Autodesk Fusion 360 part; units mm, degrees
sketch "Sketch1" plane through (0, 0, 0) normal (0, 1, 0) x (1, 0, 0)
  line L0 (0, 80) -> (-33.9737, 46.7608)
  line L1 (0, 80) -> (33.9737, 46.7608)
  line L2 (-76.0845, 24.7214) -> (-33.9737, 46.7608)
  line L3 (-76.0845, 24.7214) -> (-54.9706, -17.861)
  line L4 (-47.0228, -64.7214) -> (-54.9706, -17.861)
  line L5 (-47.0228, -64.7214) -> (0, -57.7996)
  line L6 (47.0228, -64.7214) -> (0, -57.7996)
  line L7 (47.0228, -64.7214) -> (54.9706, -17.861)
  line L8 (76.0845, 24.7214) -> (54.9706, -17.861)
  line L9 (76.0845, 24.7214) -> (33.9737, 46.7608)
  circle A0 centre (0, 0) radius 25
  dimension "d35" = 50
extrude "Extrude1" add sketch "Sketch1" along normal blind 25 contours L0 L1 L2 L3 L4 L5 L6 L7 L8 L9 | A0 makes body 1
shell "Shell1" thickness 5 outward yes removed faces 1 at (11.3246, 25, -3.6796) on bodies 1
extrude "Extrude2" add 1 faces at (-65.2553, 25, -34.1513) along direction (0, 1, 0) blind 5 separate body on bodies 1 makes body 2
extrude "Extrude3" add sketch "Sketch1" along normal blind 30 separate body contours L0 L1 L2 L3 L4 L5 L6 L7 L8 L9 | A0 makes body 3
extrude "Extrude4" cut 1 faces at (11.3246, 0, -3.6796) along direction (0, 1, 0) blind 25 on bodies 3 bodies 3
sketch "Sketch2" plane through (0, 30, 0) normal (0, 1, 0) x (-1, 0, 0)
  line L0 (-47.0228, 64.7214) -> (-54.9706, 17.861)
  line L1 (-54.9706, 17.861) -> (-76.0845, -24.7214)
  line L2 (-76.0845, -24.7214) -> (-33.9737, -46.7608)
  line L3 (-33.9737, -46.7608) -> (0, -80)
  line L4 (0, -80) -> (33.9737, -46.7608)
  line L5 (33.9737, -46.7608) -> (76.0845, -24.7214)
  line L6 (76.0845, -24.7214) -> (54.9706, 17.861)
  line L7 (54.9706, 17.861) -> (47.0228, 64.7214)
  line L8 (47.0228, 64.7214) -> (0, 57.7996)
  line L9 (0, 57.7996) -> (-47.0228, 64.7214)
  circle A0 centre (0, 0) radius 25
  dimension "d65" = 50
extrude "Extrude9" cut sketch "Sketch1" against normal blind 10 bodies 1 makes body 4 at (-6.7759, 0, 1.242)
extrude "Extrude10" cut 1 faces at (-6.7759, 0, 1.242) along direction (0, 1, 0) blind 10 on bodies 4 bodies 4
delete_body "RemoveBody1" bodies 4
extrude "Extrude14" cut sketch "Sketch2" against normal blind 5 contours A0 bodies 3
extrude "Extrude15" add sketch "Sketch2" along normal blind 5 separate body contours A0 makes body 5
shell "Shell5" thickness 2 removed faces 1 at (6.7759, 35, -1.242) on bodies 5
extrude "Extrude16" cut 1 faces at (6.7759, 30, -1.242) along direction (0, -1, 0) blind 10 on bodies 5 bodies 5
extrude "Extrude17" add 1 faces at (6.7759, 30, -1.242) along direction (0, -1, 0) blind 5 on bodies 5 bodies 3 5
combine "Combine1" operation add target body 2 tool bodies 1 3
fillet "Fillet1" radius 10 5 edges at (-51.1344, 12.5, 70.3805) (-82.7372, 12.5, -26.8829) (0, 12.5, -86.995) (82.7372, 12.5, -26.8829) (51.1344, 12.5, 70.3805) on bodies 2
extrude "Extrude18" cut 1 faces at (29.4926, -5, 63.8255) along direction (0, 1, 0) blind 5 on bodies 2 bodies 2
fillet "Fillet2" radius 10 15 edges at (56.2738, 30, 40.0786) (48.7891, 30, 67.1524) (20.7275, 30, 65.9045) (55.5066, 30, -41.1346) (78.9424, 30, -25.6499) (69.0841, 30, 0.6526) (-21.9688, 30, -65.5012) (0, 30, -83.005) (21.9688, 30, -65.5012) (-69.0841, 30, 0.6526) (-78.9424, 30, -25.6499) (-55.5066, 30, -41.1346) (-20.7275, 30, 65.9045) (-48.7891, 30, 67.1524) (-56.2738, 30, 40.0786) on bodies 2
fillet "Fillet3" radius 2.5 15 edges at (69.0841, 0, 0.6526) (78.9424, 0, -25.6499) (55.5066, 0, -41.1346) (21.9688, 0, -65.5012) (0, 0, -83.005) (-21.9688, 0, -65.5012) (-55.5066, 0, -41.1346) (-78.9424, 0, -25.6499) (-69.0841, 0, 0.6526) (-56.2738, 0, 40.0786) (-48.7891, 0, 67.1524) (-20.7275, 0, 65.9045) (20.7275, 0, 65.9045) (48.7891, 0, 67.1524) (56.2738, 0, 40.0786) on bodies 2
extrude "Extrude19" add sketch "Sketch1" along normal blind 5 separate body makes body 6
extrude "Extrude20" add sketch "Sketch1" along normal blind 5 contours A0 bodies 6
shell "Shell6" thickness 2 removed faces 1 at (11.3246, 5, -3.6796) on bodies 6
hidden bodies 6
Part model, mm, in its own coordinate system. A direction names the side the tool comes from. Round coordinates to 2 decimals unless told otherwise and drop trailing zeros. Order: outer loops, then holes, each group sorted by start corner. A loop starts at its lowest first (then second) coordinate and runs counter-clockwise, first axis right, second up. Notation, with made-up numbers: M 1.5,-5.75 L 14.5,-5.75 A17 ccw 14.5,25.25 Z; hole C -18,85 d2. An arc over 180 degrees is marked long. Answer in a Markdown table with one row per item. Add a question column.
Q1. Cut at A-A on y = 11.5. Give the cut face in (x, z).
Q2. Pin check, flat tips, straight feed: pin 1 (1.5 mm diameter, centred on x = -38, y = 24.5, fed in from +Z); pin 2 (12 mm diameter, centred on x = 16, y = 25.5, fed in from -Z); pin 3 (12 mm diameter, centred on x = -38, y = 11, fed in from -Z). Stop position of each tip, or through.
Q3. 3-axis set-ups, long thin cutter, end or side, ignore diameter. For faces 1 (the face through (20.437, 11.128, 65.862)), 2 (the face through (14, 30, 21)), 3 (the face through (-21.36, 0.71, -65.04)), 4 (the face through (55.3, 12.3, -35.6)), 5 (the face through (-20.71, 26.99, 63.02)): which of +Z, -Z, +X, -X, +Y, -Y reach the whole face in a straight line?
Q4. Mould opens along X. For faces 6 (the face through (0, 0, 58)), 7 (the face through (-16.75, 12.32, -63.61)), 8 (the face through (-20.284, 26.993, -63.16)), 9 (the face through (56.323, 11.128, 39.789)) say: +X half, -X half, draft (parallel to the pull), parting line (faces both ways), or undercut.
Q5. Wall check: L1, parallel to Z at x = 0, y = 33.1; L2, parallel to Y at x = -12, z = 14.5; L3, parallel to X at y = 11.5, z = -1. Give the ranges that are in metal, low to high. Write a range as from..to.
Established:
| question | item | result |
|---|---|---|
| 1 | outline | M -78.39,-18.12 A10 ccw -74.07,-31.42 L -36.94,-50.85 L -6.99,-80.15 A10 ccw 6.99,-80.15 L 36.94,-50.85 L 74.07,-31.42 A10 ccw 78.39,-18.12 L 59.78,19.42 L 52.77,60.73 A10 ccw 41.45,68.96 L 0,62.85 L -41.45,68.96 A10 ccw -52.77,60.73 L -59.78,19.42 Z; hole M -76.08,-24.72 L -33.97,-46.76 L 0,-80 L 33.97,-46.76 L 76.08,-24.72 L 54.97,17.86 L 47.02,64.72 L 0,57.8 L -47.02,64.72 L -54.97,17.86 Z |
| 2 | pin 1 | stops at z = 67.73 |
| 2 | pin 2 | stops at z = -76.03 |
| 2 | pin 3 | stops at z = -55.69 |
| 3 | face 1 | +Z, +Y, -Y |
| 3 | face 2 | +Y |
| 3 | face 3 | -Z, -X, -Y |
| 3 | face 4 | -Y |
| 3 | face 5 | +Z, +Y |
| 4 | face 6 | draft |
| 4 | face 7 | undercut |
| 4 | face 8 | -X half |
| 4 | face 9 | +X half |
| 5 | L1 | z = -25..-23, 23..25 |
| 5 | L2 | y = 25..32 |
| 5 | L3 | x = -69.9..-64.32, 64.32..69.9 |
